Here's how the part is built. I have some questions about the finished solid (model axes, mm). Face numbers are marked on the shaded views. A direction names the side the tool comes from. Coordinates: 2 decimals unless noted, no trailing zeros. Write each loop counter-clockwise with the first axis right and the second up, starting at its lowest first coordinate (ties: lowest second). Pieces come first, ordered by that corner, then holes.
(1) Imagine slicing it at A-A, the plane x = -20. List the corners of the cut face in (y, z) for me (3 decimals).
(2) Please list where these lines run through material, in increasing order: probe 1 along Z at (x, y) = (149.5, -71.25); probe 2 along X at (y, z) = (37, 13); probe 3 along Z at (x, y) = (126.5, 23.5) (3 decimals).
(3) Imagine slicing it at D-D, the plane z = -39.5. List the corners of the cut face in (x, y) for me (3 decimals), plus the area to 3 significant figures.
(4) Imagine slicing it at C-C, the plane x = -149.5. List the corners of the cut face in (y, z) for me (1 decimal), plus the area to 3 significant figures.
(5) Imagine slicing it at B-B, the plane z = -4. List the corners of the cut face in (x, y) for me (3 decimals).
(6) Thinking about a two-plate mould opening in Z: for the marked faces 1, 2, 3 and 4, which applies, released by +Z, released by -Z, zero draft, split by the parting line, or undercut?
(7) For pin 1 Ø7 at (x, z) = (-148, -12) entering from +Y; pin 2 Ø20.5 at (x, z) = (-20.5, 17) entering from -Y; pin 3 Ø12 at (x, y) = (92, -34.5) entering from -Z; pin 4 Ø18.5 at (x, z) = (138, -4) entering from +Y, each with a flat end and sliding along its axis, tell me the tip position at first contact or that it passes through.
(8) Which directions (+Z, -Z, +X, -X, +Y, -Y) give clear straight access to the entire face, cutting with the end or side of a thin tool? Please do the marked faces 5, 6 and 7.
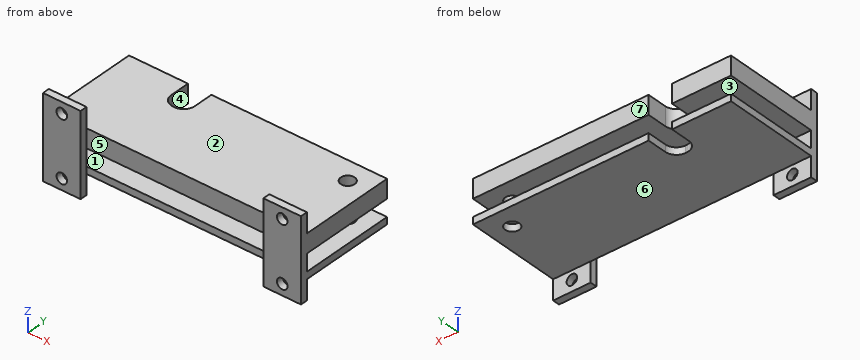
```python
from build123d import *

# Parameters (mm, degrees)
CROQUIS1_W              = 350
CROQUIS1_H              = 130
SALIENTE_EXTRUIR1_DEPTH = 29
CROQUIS2_W              = 51
CROQUIS2_H              = 112
CROQUIS2_R              = 7.14375
SALIENTE_EXTRUIR2_DEPTH = 9.525
CORTAR_EXTRUIR1_DEPTH   = 99.525
CROQUIS4_W              = 23.075
CROQUIS4_H              = 130
CORTAR_EXTRUIR2_DEPTH   = 363.201567673
CROQUIS5_R              = 9.525
CORTAR_EXTRUIR3_DEPTH   = 99.525


with BuildPart() as part:
    # Croquis1 → Saliente-Extruir1 (new, symmetric)
    with BuildSketch(Plane.XY):
        Rectangle(CROQUIS1_W, CROQUIS1_H)
    extrude(amount=SALIENTE_EXTRUIR1_DEPTH, both=True)

    # Croquis2 → Saliente-Extruir2 (add)
    # profile 1 of 2: a face of its own
    with BuildSketch(Plane.XZ.offset(65)):
        with Locations((-149.5, 0)):
            Rectangle(CROQUIS2_W, CROQUIS2_H)
        with Locations(Location((-149.5, 41.05625, 0), (0, 0, 90))):
            Circle(CROQUIS2_R, mode=Mode.SUBTRACT)
        with Locations(Location((-149.5, -41.05625, 0), (0, 0, 90))):
            Circle(CROQUIS2_R, mode=Mode.SUBTRACT)
    # profile 2 of 2: a face of its own
    with BuildSketch(Plane.XZ.offset(65)):
        with Locations((149.5, 0)):
            Rectangle(CROQUIS2_W, CROQUIS2_H)
        with Locations(Location((149.5, -41.05625, 0), (0, 0, 90))):
            Circle(CROQUIS2_R, mode=Mode.SUBTRACT)
        with Locations(Location((149.5, 41.05625, 0), (0, 0, 90))):
            Circle(CROQUIS2_R, mode=Mode.SUBTRACT)
    extrude(amount=SALIENTE_EXTRUIR2_DEPTH)

    # Croquis3 → Cortar-Extruir1 (cut)
    with BuildSketch(Plane(origin=(0, 0, -29), x_dir=(-1, 0, 0), z_dir=(0, 0, -1))):
        with BuildLine():
            Line((95, 65), (63.25, 65))
            Line((63.25, 65), (63.25, 38))
            ThreePointArc((63.25, 38), (67.643398282, 27.393398282), (78.25, 23))
            Line((78.25, 23), (80, 23))
            ThreePointArc((80, 23), (90.606601718, 27.393398282), (95, 38))
            Line((95, 38), (95, 65))
        make_face()
    extrude(amount=-CORTAR_EXTRUIR1_DEPTH, mode=Mode.SUBTRACT)

    # Croquis4 → Cortar-Extruir2 (cut, through all)
    with BuildSketch(Plane(origin=(175, 0, 0), x_dir=(0, 0, -1), z_dir=(1, 0, 0))):
        with Locations((7.9375, 0)):
            Rectangle(CROQUIS4_W, CROQUIS4_H)
    extrude(amount=-CORTAR_EXTRUIR2_DEPTH, mode=Mode.SUBTRACT)

    # Croquis5 → Cortar-Extruir3 (cut)
    with BuildSketch(Plane(origin=(0, 0, -29), x_dir=(-1, 0, 0), z_dir=(0, 0, -1))):
        with Locations((-146, 36)):
            Circle(CROQUIS5_R)
    extrude(amount=-CORTAR_EXTRUIR3_DEPTH, mode=Mode.SUBTRACT)


solid = part.part
```
Recorded:
1. outline: (-65, -29) - (65, -29) - (65, -19.475) - (-65, -19.475) - close; (-65, 3.6) - (65, 3.6) - (65, 29) - (-65, 29) - close
2. probe 1: z = -56 to -48.2, -33.91 to 33.91, 48.2 to 56
2. probe 2: x = -175 to -94.97, -63.28 to 136.53, 155.47 to 175
2. probe 3: z = -29 to -19.475, 3.6 to 29
3. outline: (-175, -74.525) - (-156.472, -74.525) - (-156.472, -65) - (-175, -65) - close; (-142.528, -74.525) - (-124, -74.525) - (-124, -65) - (-142.528, -65) - close; (124, -74.525) - (142.528, -74.525) - (142.528, -65) - (124, -65) - close; (156.472, -74.525) - (175, -74.525) - (175, -65) - (156.472, -65) - close
3. area: 706 mm2
4. outline: (-74.5, -56) - (-65, -56) - (-65, -48.2) - (-74.5, -48.2) - close; (-74.5, -33.9) - (-65, -33.9) - (-65, -29) - (65, -29) - (65, -19.5) - (-65, -19.5) - (-65, 3.6) - (65, 3.6) - (65, 29) - (-65, 29) - (-65, 33.9) - (-74.5, 33.9) - close; (-74.5, 48.2) - (-65, 48.2) - (-65, 56) - (-74.5, 56) - close
4. area: 5,330 mm2
5. outline: (-175, -74.525) - (-124, -74.525) - (-124, -65) - (-175, -65) - close; (124, -74.525) - (175, -74.525) - (175, -65) - (124, -65) - close
6. face 1: undercut
6. face 2: released by +Z
6. face 3: undercut
6. face 4: zero draft
7. pin 1: stops at y = -65
7. pin 2: stops at y = -65
7. pin 3: stops at z = -29
7. pin 4: stops at y = 65
8. face 5: +Z, -Z, -Y
8. face 6: -Z, +X, -X, +Y
8. face 7: +Z, -Z, +X, -X, +Y
